Geometry check sheet. Reference: the model listing, model coordinates, mm. A direction names the side the tool comes from. Give positions to 0.01 mm unless a question says otherwise; leave off trailing zeros. Write each loop counter-clockwise with the first axis right and the second up, starting at its lowest first coordinate (ties: lowest second). Pieces come first, ordered by that corner, then holes. Notation, with made-up numbers: (-27.75, 37.25) -> (5.25, 37.25) arc R15 ccw to (5.25, 59.25) -> close; hole circle Ø3 at (38.25, 86). An arc over 180 degrees is marked (long way). Write item = value, one per line. Start each with the question number.
1. Set-up check for faces 4 (the flat face through (18, -7, 0)), 5 (the cylindrical face through (0.056, -4.105, 1.479)): record each of +Z, -Z, +X, -X, +Y, -Y from which the full face is reachable in a straight line by a thin tool's end or side.
2. Depth check by flat-ended pin: P1, Ø2.5, axis at x = 25.08, y = -9.38, coming from the -Z side; P2, Ø1, axis at y = -3.5, z = 1, coming from the -X side; P3, Ø1.5, axis at y = -3.5, z = 1.5, coming from the +X side. Enter the tip coordinate at first touch or a pass-through.
3. Cross-section at C-C, the plane x = 7.5. Record the cut outline in (y, z).
4. Mould release check, pull along Y, two halves, no side actions. Record for faces 1 (the cylindrical face through (25.309, -17.374, 1.479)), 2 (the cylindrical face through (-0.028, -2.105, 1.479)), 3 (the flat face through (18, -7, 3)): pulls with the +Y half, pulls with the -Y half, needs draft (parallel to the pull), parting line crosses it, or undercut.
5. Cross-section at A-A, the plane y = -13. Record the cut outline in (x, z), plus the area to 3 significant figures.
6. Thickness scan on line 1 along Y through (x, z) = (-1, 1.9); line 2 along X through (y, z) = (-3.5, 1.65); line 3 along X through (y, z) = (-4, 0.65). Record the ranges inside material, lowest first.
7. Cross-section at B-B, the plane x = 16.5. Record the cut outline in (y, z).
```python
from build123d import *

# Parameters (mm, degrees)
SKETCH1_R           = 1.5
SKETCH1_R_2         = 1
BOSS_EXTRUDE1_DEPTH = 3


with BuildPart() as part:
    # Sketch1 → Boss-Extrude1 (new body)
    with BuildSketch(Plane.XY):
        with BuildLine():
            Line((0, 0), (31.010482732, 0))
            ThreePointArc((31.010482732, 0), (32.420975481, -0.582075389), (33.010455116, -1.989489797))
            Line((33.010455116, -1.989489797), (33.052571579, -10.003774465))
            ThreePointArc((33.052571579, -10.003774465), (25.143173524, -17.377139631), (17.113116724, -10.13536642))
            ThreePointArc((17.113116724, -10.13536642), (11.370616348, -8.112797173), (5.895074629, -10.774664902))
            ThreePointArc((5.895074629, -10.774664902), (-6.140954906, -10.359862027), (0, 0))
        make_face()
        with Locations((25.077129875, -9.377412246)):
            Circle(SKETCH1_R, mode=Mode.SUBTRACT)
        with Locations((29.13412022, -4.298945023)):
            Circle(SKETCH1_R_2, mode=Mode.SUBTRACT)
        with Locations((-0.375746772, -9.377412246)):
            Circle(SKETCH1_R, mode=Mode.SUBTRACT)
        with BuildLine():
            ThreePointArc((2.262283142, -5.193372604), (0.019600772, -4.104927744), (-2.237613726, -5.162906542))
            ThreePointArc((-2.237613726, -5.162906542), (-3.645044504, -5.301248889), (-3.783386851, -3.893818111))
            ThreePointArc((-3.783386851, -3.893818111), (0.033141244, -2.10497358), (3.825098224, -3.945330531))
            ThreePointArc((3.825098224, -3.945330531), (3.66771172, -5.350759109), (2.262283142, -5.193372604))
        make_face(mode=Mode.SUBTRACT)
    extrude(amount=BOSS_EXTRUDE1_DEPTH)


solid = part.part
```
Answers:
q1.face_4 = -Z, +X, -X, +Y, -Y
q1.face_5 = +Z, -Z
q2.P1 = through
q2.P2 = -6.32
q2.P3 = 33.02
q3.outline = (-9.39, 0) -> (0, 0) -> (0, 3) -> (-9.39, 3) -> close
q4.face_1 = pulls with the -Y half
q4.face_2 = undercut
q4.face_3 = needs draft
q5.outline = (-3.61, 0) -> (3.61, 0) -> (3.61, 3) -> (-3.61, 3) -> close; (17.94, 0) -> (32.21, 0) -> (32.21, 3) -> (17.94, 3) -> close
q5.area = 64.4 mm^2
q6.line_1 = -13.93 to -10.74, -8.01 to -4.28, -2.21 to -0.07
q6.line_2 = -6.06 to -3.42, 3.42 to 28.53, 29.74 to 33.02
q6.line_3 = -6.32 to -3.86, 3.87 to 28.18, 30.09 to 33.02
q7.outline = (-9.64, 0) -> (0, 0) -> (0, 3) -> (-9.64, 3) -> close
